Answer from the drawing. Dimensions are ordinates in mm from the lowest x, y and z of the part. A direction names the side the tool comes from. Round coordinates to 2 decimals unless told otherwise and drop trailing zeros. Loops run counter-clockwise (first coordinate to the right, second up) from the corner with the lowest first, then second, coordinate; pieces in that order, holes last. Notation, with made-up numbers: (-1.5, 61.5) - (9.5, 61.5) arc R31 ccw to (9.5, 94.5) - close; hole circle Ø9 at (-38, -12.5). An arc over 180 degrees is marked (long way). Write item = value, one per line. Start each with the question number.
1) Section D-D, the plane x = 20 is taken. Determine the outline of the cut face in (y, z).
2) Section B-B, the plane z = 29 is taken. Determine the outline of the cut face in (x, y).
3) A tool of negligible diameter and unlimited length cuts with its end or side. For the marked faces 5 and 6, from which of +Z, -Z, +X, -X, +Y, -Y can it reach the whole face along a straight path? Write none if from no direction.
4) Given pin 1 Ø9 at (x, z) = (35, 6) entering from +Y; pin 2 Ø3.5 at (x, z) = (6, 6.5) entering from +Y; pin 3 Ø3 at (y, z) = (26, 10) entering from -X, each flat-ended and moving along its own axis, determine where each tip first touches the part or whether it passes through.
5) Section A-A, the plane y = 15 is taken. Determine the outline of the cut face in (x, z), and give its area (3 significant figures).
6) For a pull along X with two mould halves and no side action, classify the marked faces 1, 2, 3 and 4 as released by +X, released by -X, zero draft, split by the parting line, or undercut.
7) Section C-C, the plane x = 5 is taken. Determine the outline of the cut face in (y, z), and give its area (3 significant figures).
8) Straight lines are drawn through the part: line 1 along Z through (x, y) = (35, 1.5); line 2 along Z through (x, y) = (5, 22.5); line 3 along X through (y, z) = (15, 17). For each, find the intervals that lie inside material, in ascending order.
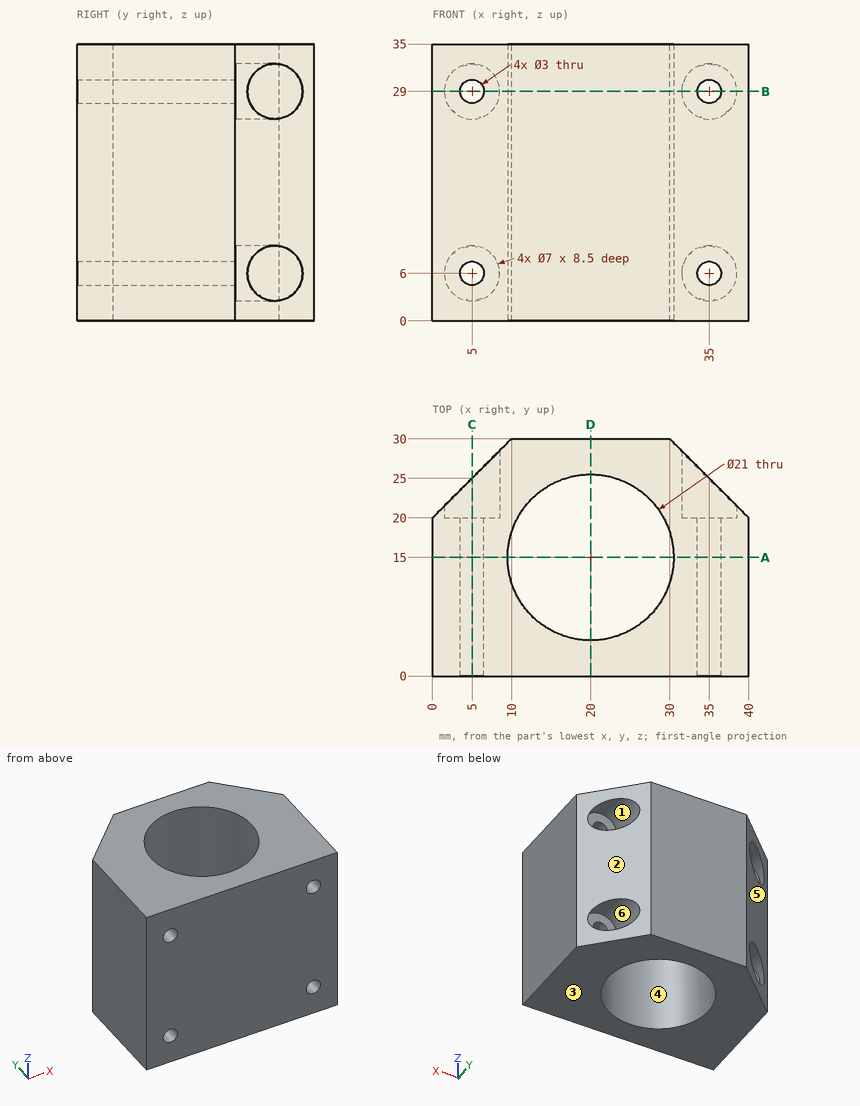
Geometry check:
q1.outline = (0, 0) - (4.5, 0) - (4.5, 35) - (0, 35) - close; (25.5, 0) - (30, 0) - (30, 35) - (25.5, 35) - close
q2.outline = (0, 0) - (3.5, 0) - (3.5, 20) - (1.5, 20) - (1.5, 21.5) - (0, 20) - close; (6.5, 0) - (33.5, 0) - (33.5, 20) - (31.5, 20) - (31.5, 28.5) - (30, 30) - (10, 30) - (8.5, 28.5) - (8.5, 20) - (6.5, 20) - close; (36.5, 0) - (40, 0) - (40, 20) - (38.5, 21.5) - (38.5, 20) - (36.5, 20) - close; hole circle Ø21 at (20, 15)
q3.face_5 = +Z, -Z, -X, +Y
q3.face_6 = +Y
q4.pin_1 = 29.5
q4.pin_2 = 20
q4.pin_3 = 4.5
q5.outline = (0, 0) - (9.5, 0) - (9.5, 35) - (0, 35) - close; (30.5, 0) - (40, 0) - (40, 35) - (30.5, 35) - close; hole circle Ø3 at (5, 6); hole circle Ø3 at (5, 29); hole circle Ø3 at (35, 6); hole circle Ø3 at (35, 29)
q5.area = 637 mm2
q6.face_1 = undercut
q6.face_2 = released by +X
q6.face_3 = zero draft
q6.face_4 = undercut
q7.outline = (0, 0) - (25, 0) - (25, 2.5) - (20, 2.5) - (20, 4.5) - (0, 4.5) - close; (0, 7.5) - (20, 7.5) - (20, 9.5) - (25, 9.5) - (25, 25.5) - (20, 25.5) - (20, 27.5) - (0, 27.5) - close; (0, 30.5) - (20, 30.5) - (20, 32.5) - (25, 32.5) - (25, 35) - (0, 35) - close
q7.area = 685 mm2
q8.line_1 = 0 to 4.5, 7.5 to 27.5, 30.5 to 35
q8.line_2 = 0 to 2.5, 9.5 to 25.5, 32.5 to 35
q8.line_3 = 0 to 9.5, 30.5 to 40
